Answer from the drawing. Dimensions are ordinates in mm from the lowest x, y and z of the part. A direction names the side the tool comes from. Give positions to 0.01 mm unless a question says otherwise; leave off trailing zeros. Write each loop counter-clockwise with the first axis right and the second up, starting at its lowest first coordinate (ties: lowest second). Pieces come first, ordered by that corner, then holes.
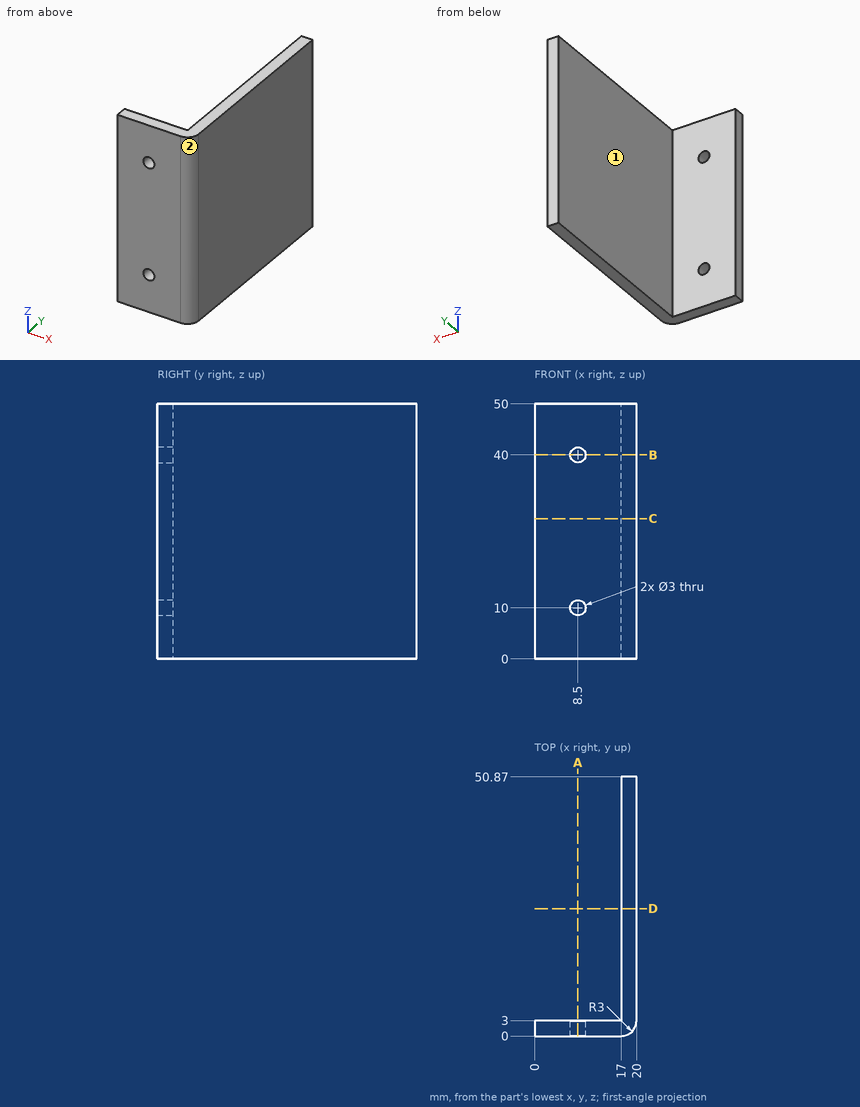
Item 1: A cutting plane is placed at A-A, the plane x = 8.5. Give the vertices of the cut face in (y, z).
Conclusion:
outline: (0, 0) - (3, 0) - (3, 8.5) - (0, 8.5) - close; (0, 11.5) - (3, 11.5) - (3, 38.5) - (0, 38.5) - close; (0, 41.5) - (3, 41.5) - (3, 50) - (0, 50) - close
Item 2: Each of these flat-tipped pins is pushed along its axis until it touches: P1, Ø14.5, axis at y = 20, z = 30, coming from the -X side; P2, Ø2, axis at x = 14.5, y = 42.5, coming from the -Z side; P3, Ø4, axis at x = 16, y = 25.5, coming from the -Z side; P4, Ø10, axis at x = 9.5, z = 19.5, coming from the +Y side. Where does it stop, or does it pass through?
Conclusion:
P1: stops at x = 17
P2: passes through
P3: stops at z = 0
P4: stops at y = 3
Item 3: Which of the six approach directions +Z, -Z, +X, -X, +Y, -Y give full straight-line access (tool end or side, diameter ignored) to the marked faces 1 and 2?
Conclusion:
face 1: +Z, -Z, -X, +Y
face 2: +Z, -Z, +X, -Y
Item 4: A cutting plane is placed at D-D, the plane y = 25. Give the vertices of the cut face in (x, z).
Conclusion:
outline: (17, 0) - (20, 0) - (20, 50) - (17, 50) - close
Item 5: A cutting plane is placed at C-C, the plane z = 27.5. Give the vertices of the cut face in (x, y), plus the area to 3 significant figures.
Conclusion:
outline: (0, 0) - (17, 0) arc R3 ccw to (20, 3) - (20, 50.87) - (17, 50.87) - (17, 3) - (0, 3) - close
area: 202 mm2
Item 6: Consider probe 1 along X at (y, z) = (45.5, 21); probe 2 along X at (y, z) = (1.4, 40); probe 3 along Y at (x, z) = (11.25, 20). Determine where each line is inside the solid, lowest interval first.
Conclusion:
probe 1: x = 17 to 20
probe 2: x = 0 to 7, 10 to 19.54
probe 3: y = 0 to 3
Item 7: A cutting plane is placed at B-B, the plane z = 40. Give the vertices of the cut face in (x, y).
Conclusion:
outline: (0, 0) - (7, 0) - (7, 3) - (0, 3) - close; (10, 0) - (17, 0) arc R3 ccw to (20, 3) - (20, 50.87) - (17, 50.87) - (17, 3) - (10, 3) - close
